Design review of the part built by this model. Coordinates are the model's own, in mm. Face numbers are marked on the shaded views. Give positions to 0.01 mm unless a question says otherwise; leave off trailing zeros. Loops run counter-clockwise (first coordinate to the right, second up) from the corner with the lowest first, then second, coordinate; pieces in that order, holes last.
from build123d import *

# Parameters (mm, degrees)
F0_R     = 127.208159
F1_DEPTH = 381
F2_R     = 27.237413
F3_DEPTH = 50.8
F4_R     = 12.7
F5_R     = 12.7


with BuildPart() as f1:
    # F0 (on Front) → F1 (new body)
    with BuildSketch(Plane.XZ):
        Circle(F0_R)
    extrude(amount=F1_DEPTH)

    # F2 (on face) → F3 (cut)
    with BuildSketch(Plane.XZ.offset(381)):
        with Locations((0, 10.933507)):
            Circle(F2_R)
    extrude(amount=-F3_DEPTH, mode=Mode.SUBTRACT)

    # F4
    f4_edges = [f1.edges().sort_by_distance(p)[0] for p in [
        (-127.208159, -381, 0),
    ]]
    fillet(f4_edges, radius=F4_R)

    # F5
    f5_edges = [f1.edges().sort_by_distance(p)[0] for p in [
        (-127.208159, 0, 0),
    ]]
    fillet(f5_edges, radius=F5_R)


solid = f1.part
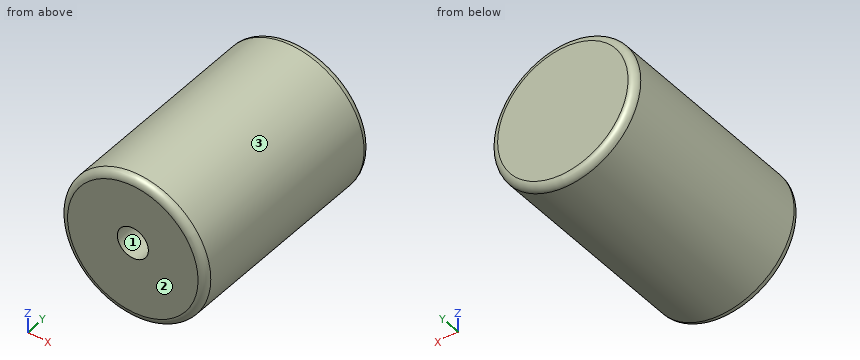
Q1. Insertion check: pin 1 (3 mm diameter, centred on x = 52.5, y = -290, fed in from +Z); pin 2 (3 mm diameter, centred on x = 76, y = -86.5, fed in from -Z); pin 3 (16.5 mm diameter, centred on x = -13, z = 18, fed in from -Y). Each pin has a flat end and moves straight along its axis. Give the tip position at first contact, or say it passes through.
Results:
pin 1: stops at z = 116.54
pin 2: stops at z = -103.11
pin 3: stops at y = -330.2
Q2. Wall thickness on line 1 (Z direction, x = 0, y = -360); line 2 (X direction, y = -243.5, z = -3.5); line 3 (Z direction, x = 50.5, y = -301): over which ranges is each line inside the solid? List them lowest first.
Results:
line 1: z = -127.21 to -16.3, 38.17 to 127.21
line 2: x = -127.16 to 127.16
line 3: z = -116.75 to 116.75
Q3. Draft analysis for pull direction X (two halves, no side actions). For the marked faces 1, 2 and 3, state which applies: pulls with the +X half, pulls with the -X half, needs draft (parallel to the pull), parting line crosses it, or undercut.
Results:
face 1: undercut
face 2: needs draft
face 3: parting line crosses it
Q4. Take a section at B-B (z = 0). Give the boundary of the cut face in (x, y).
Results:
outline: (-127.21, -368.3) arc R12.7 ccw to (-114.51, -381) - (-24.95, -381) - (-24.95, -330.2) - (24.95, -330.2) - (24.95, -381) - (114.51, -381) arc R12.7 ccw to (127.21, -368.3) - (127.21, -12.7) arc R12.7 ccw to (114.51, 0) - (-114.51, 0) arc R12.7 ccw to (-127.21, -12.7) - close
Q5. Take a section at A-A (x = 0). Give the boundary of the cut face in (y, z), plus the area to 3 significant figures.
Results:
outline: (-381, -114.51) arc R12.7 ccw to (-368.3, -127.21) - (-12.7, -127.21) arc R12.7 ccw to (0, -114.51) - (0, 114.51) arc R12.7 ccw to (-12.7, 127.21) - (-368.3, 127.21) arc R12.7 ccw to (-381, 114.51) - (-381, 38.17) - (-330.2, 38.17) - (-330.2, -16.3) - (-381, -16.3) - close
area: 94,000 mm2
Q6. Take a section at C-C (y = -77). Give the boundary of the cut face in (x, z).
Results:
outline: circle Ø254.42 at (0, 0)
